Read the model definition and answer for the solid it produces. Units are mm, in the model's axes. A direction names the side the tool comes from. Give positions to 0.01 mm unless a question says otherwise; leave off trailing zeros. Loops run counter-clockwise (first coordinate to the right, second up) from the corner with the lowest first, then second, coordinate; pieces in that order, holes last. Notation, with made-up numbers: (0, -29.75) - (31, -29.75) arc R32 ccw to (31, 0.25) - close; hole circle Ø8 at (41, 69). An arc over 180 degrees is marked (long way). Write item = value, one per line.
Autodesk Inventor part; units mm, degrees
ref_plane "YZ Plane" through (0, 0, 0) normal (1, 0, 0) x (0, 1, 0)
ref_plane "XZ Plane" through (0, 0, 0) normal (0, 1, 0) x (-1, 0, 0)
ref_plane "XY Plane" through (0, 0, 0) normal (0, 0, 1) x (1, 0, 0)
sketch "Sketch1" plane through (0, 0, 0) normal (0, 0, 1) x (1, 0, 0)
  line L0 (2.8868, 0) -> (1.4434, -2.5)
  line L1 (1.4434, -2.5) -> (-1.4434, -2.5)
  line L2 (-1.4434, -2.5) -> (-2.8868, 0)
  line L3 (-2.8868, 0) -> (-1.4434, 2.5)
  line L4 (-1.4434, 2.5) -> (1.4434, 2.5)
  line L5 (1.4434, 2.5) -> (2.8868, 0)
  point P0 (0, 0)
  point P1 (0, 0)
  dimension "d0" = 5
extrude "Extrusion1" add sketch "Sketch1" along normal blind 5
sketch "Sketch2" plane through (0, 0, 5) normal (0, 0, 1) x (1, 0, 0)
  circle A0 centre (0, 0) radius 1.5
  dimension "d3" = 3
extrude "Extrusion2" add sketch "Sketch2" along normal blind 4
chamfer "Chamfer1" distance 0.5 angle 45 1 edges at (-1.5, 0, 9)
thread "Thread1"
sketch "Sketch3" plane through (0, 0, 0) normal (0, 0, -1) x (-1, 0, 0)
  point P0 (0, 0)
  point P1 (0, 0)
hole "Hole1" at (0, 0, 0) direction (0, 0, 1) diameter 2.459 depth 4 tip angle 118
properties part number "Abstandshalter_5mm" material "Stainless Steel"
1) A tool of negligible diameter and unlimited length cuts with its end or side. For faces 1 (the face through (-1.5, -0.07, 6.73)), 2 (the face through (2.175, -1.233, 2.465)), from which of +Z, -Z, +X, -X, +Y, -Y can it reach the whole face along a straight path? Write none if from no direction.
Output:
face_1 = +Z
face_2 = +Z, -Z, +X, -Y
2) Find the intervals of material crossed by probe 1 along Y at (x, z) = (0, 2); probe 2 along Z at (x, y) = (2.1, -0.7); probe 3 along X at (y, z) = (-0.85, 0.5), in increasing order.
Output:
probe_1 = -2.5 to -1.23, 1.23 to 2.5
probe_2 = 0 to 5
probe_3 = -2.4 to -0.89, 0.89 to 2.4
3) A cutting plane is placed at A-A on z = 2. Determine the outline of the cut face in (x, y).
Output:
outline = (-2.89, 0) - (-1.44, -2.5) - (1.44, -2.5) - (2.89, 0) - (1.44, 2.5) - (-1.44, 2.5) - close; hole circle Ø2.46 at (0, 0)
4) A cutting plane is placed at B-B on z = 4.5. Determine the outline of the cut face in (x, y), then the cut area to 3 significant figures.
Output:
outline = (-2.89, 0) - (-1.44, -2.5) - (1.44, -2.5) - (2.89, 0) - (1.44, 2.5) - (-1.44, 2.5) - close; hole circle Ø0.79 at (0, 0)
area = 21.2 mm²
5) A cutting plane is placed at D-D on y = 2.05. Determine the outline of the cut face in (x, z).
Output:
outline = (-1.7, 0) - (1.7, 0) - (1.7, 5) - (-1.7, 5) - close
6) A cutting plane is placed at C-C on z = 8. Determine the outline of the cut face in (x, y).
Output:
outline = circle Ø3 at (0, 0)
7) The mould has two halves that part along Y. Classify faces 3 (the face through (-2.175, 1.233, 2.465)), 4 (the face through (0.064, 0.204, 4.61)), 5 (the face through (0.748, -0.976, 2.028)), 6 (the face through (0, -2.5, 2)): pulls with the +Y half, pulls with the -Y half, needs draft (parallel to the pull), parting line crosses it, or undercut.
Output:
face_3 = pulls with the +Y half
face_4 = undercut
face_5 = undercut
face_6 = pulls with the -Y half
